Here's how the part is built. I have some questions about the finished solid (model axes, mm). A direction names the side the tool comes from. Coordinates: 2 decimals unless noted, no trailing zeros. Loops run counter-clockwise (first coordinate to the right, second up) from the corner with the lowest first, then second, coordinate; pieces in that order, holes last.
Autodesk Inventor part; units mm, degrees
ref_plane "YZ Plane" through (0, 0, 0) normal (1, 0, 0) x (0, 1, 0)
ref_plane "XZ Plane" through (0, 0, 0) normal (0, 1, 0) x (-1, 0, 0)
ref_plane "XY Plane" through (0, 0, 0) normal (0, 0, 1) x (1, 0, 0)
sketch "スケッチ3" plane through (0, 0, 0) normal (0, 1, 0) x (-1, 0, 0)
  line L0 (0, 0) -> (5, 0)
  line L1 (5, 0) -> (5, 10)
  line L2 (5, 10) -> (0, 10)
  line L3 (0, 10) -> (0, 0)
  line L4 (0, 6) -> (-4, 6)
  line L5 (-4, 6) -> (-4, 4)
  line L6 (-4, 4) -> (0, 4)
  line L7 (0, 4) -> (0, 6)
  line L8 (-4, 25) -> (-39, 25)
  line L9 (-39, 25) -> (-39, -15)
  line L10 (-39, -15) -> (-4, -15)
  line L11 (-4, -15) -> (-4, 25)
  point P0 (0, 5)
  point P1 (0, 4)
  dimension "d5" = 5
  dimension "d6" = 10
  dimension "d7" = 4
  dimension "d8" = 2
  dimension "d9" = 35
  dimension "d10" = 4
  dimension "d11" = 40
  dimension "d12" = 20
extrude "押し出し2" add sketch "スケッチ3" along normal blind 10 and the other way blind 30 contours L3 L2 L1 L0
extrude "押し出し3" [suppressed]
sketch "スケッチ4" plane through (-5, -30, 10) normal (-1, 0, 0) x (0, 0, 1)
  line L0 (0, 38.8506) -> (-2.25, 39.6696)
  line L1 (0, 0) -> (0, 40)
  line L2 (0, 38.0078) -> (-2.25, 37.1888)
  line L3 (-10, 40) -> (0, 40)
  line L4 (0, 38.4292) -> (-2.25, 38.4292)
  line L5 (0, 40) -> (-10, 40)
  line L6 (-1, 40) -> (-1, 36.8584)
  line L7 (-2.25, 40) -> (-2.25, 36.8584)
  line L8 (0, 36.8584) -> (-2.25, 36.8584)
  line L9 (-1, 40) -> (-1, 39.2146)
  line L10 (-1, 39.2146) -> (-1, 38.4292)
  line L11 (-1, 38.4292) -> (-1, 37.6438)
  line L12 (-1, 37.6438) -> (-1, 36.8584)
  point P0 (-10, 30)
  dimension "d21" = 20
  dimension "d23" = 1
  dimension "d24" = 1.25
  dimension "d25" = 1.5708
  dimension "d27" = 1.5708
  dimension "d28" = 20
extrude "押し出し4" cut sketch "スケッチ4" against normal blind 5 contours L0 L6 L3 L1 | L0 L7 L3 L6 | L1 L8 L6 L2 | L6 L8 L7 L2
fillet "フィレット1" radius 0.3 2 edges at (-2.5, 9.6696, 7.75) (-2.5, 7.1888, 7.75)
chamfer "面取り1" distance 0.1 angle 45 2 edges at (-2.5, 8.8506, 10) (-2.5, 8.0078, 10)
pattern_linear "矩形状パターン1" count 10 spacing 3.1416 along (0, -1, 0) of "押し出し4", "フィレット1", "面取り1"
sketch "スケッチ5" plane through (-5, -30, 0) normal (-1, 0, 0) x (0, 0, 1)
  line L0 (10, 8.5841) -> (10, 0)
  line L1 (10, 8.5841) -> (0, 8.5841)
  line L2 (0, 8.5841) -> (0, 0)
  line L3 (0, 0) -> (10, 0)
  line L4 (10, 0) -> (10, 8.5841)
  point P0 (0, 30)
extrude "押し出し5" cut sketch "スケッチ5" against normal blind 10
equation "\"d23\" = module"
equation "\"d24\" = 1.25 * module"
equation "\"d25\" = 1.5708 * module"
equation "\"d27\" = d25"
equation "\"d28\" = d21"
equation "\"d37\" = 3.14159 * module"
equation "\"module\" = 1"
properties part number "tume"
Q1. Suppose I cut it at A-A on z = 8.25. State how many separate pieces and enclosed holes the cut face has, and give its area (3 significant figures).
Q2. Suppose I cut it at B-B on y = -17.5. Write out the boundary of the cut face in (x, z).
Q3. Please list where these lines run through material, in increasing order: probe 1 along Z at (x, y) = (-1.35, -9); probe 2 along Z at (x, y) = (-2.3, -10).
Q4. We'd pull the mould along Y, two halves only. Please class faces 3 (the flat face through (-2.535, -15.897, 8.94)), 4 (the flat face through (-2.535, 9.236, 8.94)), 5 (the flat face through (-3, -21.416, 4)): pulls with the +Y half, pulls with the -Y half, needs draft (parallel to the pull), parting line crosses it, or undercut.
Q5. For faces 1 (the flat face through (-2.54, -19.04, 8.94)), 2 (the flat face through (-2, -6, 0)), which set-ups out of +Z, -Z, +X, -X, +Y, -Y let a thin tool reach every point of the face, with its end or its side?
Check values:
1. separate pieces: 10
1. enclosed holes: 0
1. area: 106 mm2
2. outline: (-5, 0) - (0, 0) - (0, 8.97) - (-5, 8.97) - close
3. probe 1: z = 0 to 7.75
3. probe 2: z = 0 to 9.93
4. face 3: undercut
4. face 4: pulls with the +Y half
4. face 5: pulls with the -Y half
5. face 1: +Z, +X, -X
5. face 2: -Z, +X, -X, +Y, -Y
